Design review of the part built by this model. Coordinates are the model's own, in mm. Face numbers are marked on the shaded views. A direction names the side the tool comes from. Give positions to 0.01 mm unless a question says otherwise; leave off trailing zeros. Write each loop counter-clockwise with the first axis right and the second up, starting at its lowest first coordinate (ties: lowest second). Pieces come first, ordered by that corner, then holes. Notation, with made-up numbers: M 82.5,72 L 93.5,72 A30 ccw 93.5,108 Z; hole C 45,65 d2. An arc over 180 degrees is marked long. One line per item, written item: value. Start each with the question number.
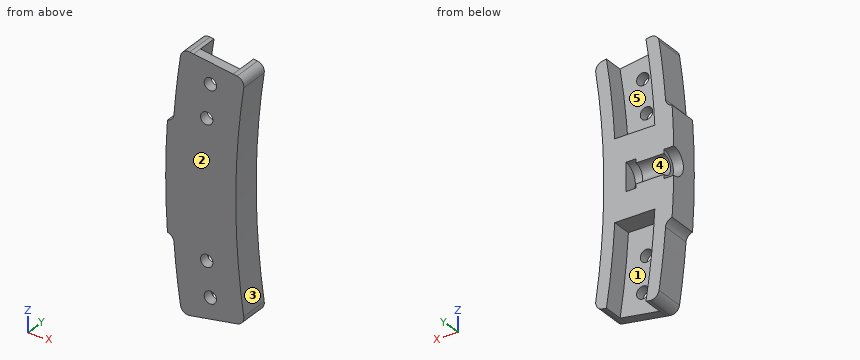
```python
from build123d import *

# Parameters (mm, degrees)
BOSS_EXTRUDE1_DEPTH        = 7.5
BOSS_EXTRUDE2_DEPTH        = 7.5
CUT_EXTRUDE1_DEPTH         = 5
F_3_1_3_1_DIAMETER_HOLE2_D = 3.1
SKETCH21_R                 = 3.5
CUT_EXTRUDE2_DEPTH         = 2.5
CUT_EXTRUDE3_START         = 2.5
SKETCH23_R                 = 3.5
CUT_EXTRUDE3_DEPTH         = 2.5
SKETCH22_R                 = 2.5
CUT_EXTRUDE4_DEPTH         = 35.217583069
FILLET1_R                  = 2
FILLET2_R                  = 2


with BuildPart() as part:
    # Sketch1 → Boss-Extrude1 (new body)
    with BuildSketch(Plane(origin=(0, 0, 0), x_dir=(1, 0, 0), z_dir=(0, 1, 0))):
        with BuildLine():
            ThreePointArc((-187.660784713, 29.722548358), (-190, 0), (-187.660784713, -29.722548358))
            Line((-187.660784713, -29.722548358), (-197.537668119, -31.286893008))
            ThreePointArc((-197.537668119, -31.286893008), (-200, 0), (-197.537668119, 31.286893008))
            Line((-197.537668119, 31.286893008), (-187.660784713, 29.722548358))
        make_face()
        with BuildLine():
            ThreePointArc((-197.537668119, -31.286893008), (-200, 0), (-197.537668119, 31.286893008))
            Line((-197.537668119, 31.286893008), (-200.500733141, 31.756196403))
            ThreePointArc((-200.500733141, 31.756196403), (-203, 0), (-200.500733141, -31.756196403))
            Line((-200.500733141, -31.756196403), (-197.537668119, -31.286893008))
        make_face()
        with BuildLine():
            Line((-184.697719691, 29.253244963), (-187.660784713, 29.722548358))
            ThreePointArc((-187.660784713, 29.722548358), (-190, 0), (-187.660784713, -29.722548358))
            Line((-187.660784713, -29.722548358), (-184.697719691, -29.253244963))
            ThreePointArc((-184.697719691, -29.253244963), (-187, 0), (-184.697719691, 29.253244963))
        make_face()
    extrude(amount=BOSS_EXTRUDE1_DEPTH)

    # Sketch19 → Boss-Extrude2 (add)
    with BuildSketch(Plane(origin=(0, 0, 0), x_dir=(1, 0, 0), z_dir=(0, 1, 0))):
        with BuildLine():
            Line((-204.062149802, 13.374939928), (-202.565361417, 13.276835234))
            ThreePointArc((-202.565361417, 13.276835234), (-203, 0), (-202.565361417, -13.276835234))
            Line((-202.565361417, -13.276835234), (-204.062149802, -13.374939928))
            ThreePointArc((-204.062149802, -13.374939928), (-204.5, 0), (-204.062149802, 13.374939928))
        make_face()
    extrude(amount=BOSS_EXTRUDE2_DEPTH)

    # Sketch15 → Cut-Extrude1 (cut)
    with BuildSketch(Plane(origin=(0, 7.5, 0), x_dir=(1, 0, 0), z_dir=(0, 1, 0))):
        with BuildLine():
            Line((-199.749843554, 10), (-189.73665961, 10))
            ThreePointArc((-189.73665961, 10), (-188.956218405, 19.88837666), (-187.660784713, 29.722548358))
            Line((-187.660784713, 29.722548358), (-197.537668119, 31.286893008))
            ThreePointArc((-197.537668119, 31.286893008), (-198.928692466, 20.673057674), (-199.749843554, 10))
        make_face()
        with BuildLine():
            ThreePointArc((-187.660784713, -29.722548358), (-188.956218405, -19.88837666), (-189.73665961, -10))
            Line((-189.73665961, -10), (-199.749843554, -10))
            ThreePointArc((-199.749843554, -10), (-198.928692466, -20.673057674), (-197.537668119, -31.286893008))
            Line((-197.537668119, -31.286893008), (-187.660784713, -29.722548358))
        make_face()
    extrude(amount=-CUT_EXTRUDE1_DEPTH, mode=Mode.SUBTRACT)

    # Ø3.1 (3.1) Diameter Hole2 (through all)
    with Locations(Plane(origin=(0, 0, 0), x_dir=(-1, 0, 0), z_dir=(0, -1, 0))):
        with Locations((193.331747968, -25.452607483), (194.257966128, -16.995369836), (194.257966128, 16.995369836), (193.331747968, 25.452607483)):
            Hole(F_3_1_3_1_DIAMETER_HOLE2_D / 2)

    # Sketch21 → Cut-Extrude2 (cut)
    with BuildSketch(Plane(origin=(-192.5, 0, 0), x_dir=(0, 0, -1), z_dir=(1, 0, 0))):
        with Locations((0, 7.5)):
            Circle(SKETCH21_R)
    extrude(amount=-CUT_EXTRUDE2_DEPTH, mode=Mode.SUBTRACT)

    # Sketch23 → Cut-Extrude3 (cut)
    with BuildSketch(Plane(origin=(-204.5, 0, 0), x_dir=(0, 0, -1), z_dir=(1, 0, 0)).offset(CUT_EXTRUDE3_START)):
        with Locations((0, 7.5)):
            Circle(SKETCH23_R)
    extrude(amount=-CUT_EXTRUDE3_DEPTH, mode=Mode.SUBTRACT)

    # Sketch22 → Cut-Extrude4 (cut, through all)
    with BuildSketch(Plane(origin=(-195, 0, 0), x_dir=(0, 0, -1), z_dir=(1, 0, 0))):
        with Locations((0, 7.5)):
            Circle(SKETCH22_R)
    extrude(amount=-CUT_EXTRUDE4_DEPTH, mode=Mode.SUBTRACT)

    # Fillet1
    fillet1_edges = [part.edges().sort_by_distance(p)[0] for p in [
        (-200.500733141, 3.75, 31.756196403),
        (-200.500733141, 3.75, -31.756196403),
        (-184.697719691, 3.75, -29.253244963),
        (-184.697719691, 3.75, 29.253244963),
    ]]
    fillet(fillet1_edges, radius=FILLET1_R)

    # Fillet2
    # the kernel refuses this fillet: 2 mm, written as the material it adds along each edge
    with BuildSketch(Plane(origin=(-202.565361417, 0, -13.276835234), x_dir=(0.0701211938680431, 0, -0.9975384795437819), z_dir=(0, 1, 0))) as fillet2_piece_1:
        with BuildLine():
            CenterArc((1.929399735, 1.999977637), FILLET2_R, 194.477346772, 75.251705008)
            Line((-0.007093381, 1.499983228), (-0.045823244, 1.48998334))
            ThreePointArc((-0.045823244, 1.48998334), (-0.043546243, 0.749802457), (-0.039999553, -0.000189157))
            Line((-0.039999553, -0.000189157), (0.000189157, -0.039999553))
            ThreePointArc((0.000189157, -0.039999553), (0.959970947, -0.037730174), (1.919752737, -0.039999553))
            Line((1.919752737, -0.039999553), (1.919941893, 0))
        make_face()
    extrude(amount=7.5)
    with BuildSketch(Plane(origin=(-202.565361417, 0, 13.276835234), x_dir=(-0.9978589232386035, 0, 0.06540312923014294), z_dir=(0, 1, 0))) as fillet2_piece_2:
        with BuildLine():
            CenterArc((1.990831296, 1.938835898), FILLET2_R, 180.54189644, 75.251705008)
            Line((-0.009079253, 1.919920426), (-0.049077464, 1.919542116))
            ThreePointArc((-0.049077464, 1.919542116), (-0.042269379, 0.95978179), (-0.04, 0))
            Line((-0.04, 0), (0, -0.04))
            ThreePointArc((0, -0.04), (0.75, -0.04), (1.490183374, -0.038776718))
            Line((1.490183374, -0.038776718), (1.5, 0))
        make_face()
    extrude(amount=7.5)


solid = part.part
```
Q1. Wall thickness on line 1 (Y direction, x = -191.5, z = -18); line 2 (X direction, y = 3.5, z = -22); line 3 (X direction, y = 2.25, z = 16): over which ranges is each line inside the solid? List them lowest first. Write a range as from..to.
Q2. Take a section at C-C, the plane y = 1.75. Give the boundary of the cut face in (x, z), then the cut area to 3 significant figures.
Q3. For P1, Ø1.5, axis at x = -194, y = 5, coming from the +Z side; P2, Ø3.5, axis at x = -193.33, z = 25.45, coming from the +Y side; P3, Ø4, axis at x = -193.5, y = 5.5, coming from the -Z side, all flat-tipped, find the tip position at first contact; note any pin that passes through.
Q4. Take a section at A-A, the plane z = 0. Give the boundary of the cut face in (x, y).
Q5. Take a section at B-B, the plane x = -193.75. Give the boundary of the cut face in (y, z).
Q6. Machinability: for the marked faces 1 and 2, which of the approach directions +Z, -Z, +X, -X, +Y, -Y give a long, thin tool a straight path to every point of the face, cutting with its end or side? Answer none if there is none.
Q7. The part is to be moulded in two halves that separate along X. For the marked faces 3, 4 and 5, say which applies: pulls with the +X half, pulls with the -X half, needs draft (parallel to the pull), parting line crosses it, or undercut.
Results list:
1. line 1: y = 0..2.5
1. line 2: x = -201.8..-198.79, -188.72..-185.7
1. line 3: x = -202.37..-195.45, -193.07..-186.31
2. outline: M -204.06,-13.37 A2 cw -202.43,-15.19 A203 ccw -200.81,-29.76 A2 ccw -198.52,-31.44 L -186.66,-29.56 A2 ccw -185,-27.3 A187 cw -185,27.3 A2 ccw -186.66,29.56 L -198.52,31.44 A2 ccw -200.81,29.76 A203 ccw -202.43,15.19 A2 cw -204.06,13.37 A204.5 ccw Z; hole C -194.26,-17 d3.1; hole C -194.26,17 d3.1; hole C -193.33,-25.45 d3.1; hole C -193.33,25.45 d3.1
2. area: 988 mm^2
3. P1: stops at z = 10
3. P2: stops at y = 2.5
3. P3: stops at z = -10
4. outline: M -204.5,0 L -187,0 L -187,7.5 L -192.5,7.5 L -192.5,4 L -195,4 L -195,5 L -202,5 L -202,4 L -204.5,4 Z
5. outline: M 0,-30.69 L 2.5,-30.69 L 2.5,-26.95 L 0,-26.95 Z; M 0,-23.96 L 2.5,-23.96 L 2.5,-18.46 L 0,-18.46 Z; M 0,-15.53 L 2.5,-15.53 L 2.5,-10 L 7.5,-10 L 7.5,-3.5 A3.5 cw 7.5,3.5 L 7.5,10 L 2.5,10 L 2.5,15.53 L 0,15.53 Z; M 0,18.46 L 2.5,18.46 L 2.5,23.96 L 0,23.96 Z; M 0,26.95 L 2.5,26.95 L 2.5,30.69 L 0,30.69 Z
6. face 1: +Y
6. face 2: +Z, -Z, +X, -X, -Y
7. face 3: pulls with the +X half
7. face 4: needs draft
7. face 5: undercut
